Autodesk Inventor part; units mm, degrees
ref_plane "YZ Plane" through (0, 0, 0) normal (1, 0, 0) x (0, 1, 0)
ref_plane "XZ Plane" through (0, 0, 0) normal (0, 1, 0) x (-1, 0, 0)
ref_plane "XY Plane" through (0, 0, 0) normal (0, 0, 1) x (1, 0, 0)
sketch "Sketch1" plane through (0, 0, 0) normal (0, 0, 1) x (1, 0, 0)
  line L0 (40.11, 59.8927) -> (-34.89, 59.8927)
  line L1 (-34.89, 59.8927) -> (-34.89, -60.1073)
  line L2 (-34.89, -60.1073) -> (40.11, -60.1073)
  line L3 (-52.89, 89.8927) -> (68.11, 89.8927)
  line L4 (68.11, -90.1073) -> (-52.89, -90.1073)
  line L5 (-64.89, -78.1073) -> (-64.89, 77.8927)
  line L6 (80.11, 47.3927) -> (91.11, 47.3927)
  line L7 (95.11, 43.3927) -> (95.11, 36.3927)
  line L8 (91.11, 32.3927) -> (80.11, 32.3927)
  line L9 (115.11, -0.1073) -> (-34.89, -0.1073) construction
  line L10 (80.11, -47.6073) -> (91.11, -47.6073)
  line L11 (95.11, -43.6073) -> (95.11, -36.6073)
  line L12 (91.11, -32.6073) -> (80.11, -32.6073)
  line L13 (80.11, 77.8927) -> (80.11, 47.3927)
  line L14 (80.11, -47.6073) -> (80.11, -78.1073)
  arc A0 (95.11, 43.3927) -> (91.11, 47.3927) centre (91.11, 43.3927) ccw
  arc A1 (91.11, 32.3927) -> (95.11, 36.3927) centre (91.11, 36.3927) ccw
  arc A2 (95.11, -36.6073) -> (91.11, -32.6073) centre (91.11, -36.6073) ccw
  arc A3 (91.11, -47.6073) -> (95.11, -43.6073) centre (91.11, -43.6073) ccw
  arc A4 (80.11, 77.8927) -> (68.11, 89.8927) centre (68.11, 77.8927) ccw
  arc A5 (68.11, -90.1073) -> (80.11, -78.1073) centre (68.11, -78.1073) ccw
  arc A6 (-64.89, -78.1073) -> (-52.89, -90.1073) centre (-52.89, -78.1073) ccw
  arc A7 (-52.89, 89.8927) -> (-64.89, 77.8927) centre (-52.89, 77.8927) ccw
  line L15 (44.11, 19.8927) -> (76.11, 19.8927)
  line L16 (76.11, -20.1073) -> (44.11, -20.1073)
  line L17 (80.11, 32.3927) -> (80.11, 23.8927)
  line L18 (80.11, -24.1073) -> (80.11, -32.6073)
  line L19 (40.11, -60.1073) -> (40.11, -24.1073)
  line L20 (40.11, 23.8927) -> (40.11, 59.8927)
  arc A8 (76.11, 19.8927) -> (80.11, 23.8927) centre (76.11, 23.8927) ccw
  arc A9 (40.11, 23.8927) -> (44.11, 19.8927) centre (44.11, 23.8927) ccw
  arc A10 (44.11, -20.1073) -> (40.11, -24.1073) centre (44.11, -24.1073) ccw
  arc A11 (80.11, -24.1073) -> (76.11, -20.1073) centre (76.11, -24.1073) ccw
  line L21 (211.9676, -294.2124) -> (139.9676, -294.2124)
  line L22 (135.9676, -414.2124) -> (215.9676, -414.2124)
  line L23 (139.9676, -334.2124) -> (211.9676, -334.2124)
  line L24 (215.9676, -374.2124) -> (135.9676, -374.2124)
  line L25 (215.9676, -414.2124) -> (215.9676, -374.2124)
  line L26 (135.9676, -298.2124) -> (135.9676, -330.2124)
  line L27 (135.9676, -374.2124) -> (135.9676, -414.2124)
  line L28 (226.9676, -306.7124) -> (215.9676, -306.7124)
  line L29 (215.9676, -321.7124) -> (226.9676, -321.7124)
  line L30 (230.9676, -317.7124) -> (230.9676, -310.7124)
  line L31 (215.9676, -330.2124) -> (215.9676, -321.7124)
  line L32 (215.9676, -306.7124) -> (215.9676, -298.2124)
  arc A12 (230.9676, -310.7124) -> (226.9676, -306.7124) centre (226.9676, -310.7124) ccw
  arc A13 (226.9676, -321.7124) -> (230.9676, -317.7124) centre (226.9676, -317.7124) ccw
  arc A14 (211.9676, -334.2124) -> (215.9676, -330.2124) centre (211.9676, -330.2124) ccw
  arc A15 (135.9676, -330.2124) -> (139.9676, -334.2124) centre (139.9676, -330.2124) ccw
  arc A16 (139.9676, -294.2124) -> (135.9676, -298.2124) centre (139.9676, -298.2124) ccw
  arc A17 (215.9676, -298.2124) -> (211.9676, -294.2124) centre (211.9676, -298.2124) ccw
  point P0 (95.11, 32.3927)
  point P1 (95.11, 47.3927)
  point P2 (87.61, 39.8927)
  point P3 (87.61, -40.1073)
  point P4 (95.11, -32.6073)
  point P5 (95.11, -47.6073)
  point P6 (87.61, -40.1073)
  point P7 (135.9676, -294.2124)
  point P8 (135.9676, -334.2124)
  point P9 (230.9676, -306.7124)
  dimension "d22" = 75
  dimension "d23" = 120
  dimension "d24" = 30
  dimension "d25" = 15
  dimension "d26" = 15
  dimension "d27" = 80
  dimension "d28" = 4
  dimension "d29" = 4
  dimension "d30" = 12
  dimension "d31" = 40
  dimension "d32" = 4
  dimension "d33" = 7.5
  dimension "d34" = 7.5
  dimension "d52" = 80
  dimension "d53" = 120
  dimension "d54" = 40
  dimension "d55" = 40
  dimension "d56" = 15
  dimension "d58" = 15
  dimension "d59" = 12.5
  dimension "d60" = 12.5
  dimension "d61" = 4
  dimension "d62" = 40
  dimension "d63" = 15
extrude "Extrusion1" add sketch "Sketch1" along normal blind 5 contours L0 L1 L2 L19 A10 L16 A11 L18 L12 A2 L11 A3 L10 L14 A5 L4 A6 L5 A7 L3 A4 L13 L6 A0 L7 A1 L8 L17 A8 L15 A9 L20
sketch "Sketch3" plane through (0, 0, 5) normal (0, 0, 1) x (1, 0, 0)
  line L0 (95.11, 36.3927) -> (95.11, 43.3927)
  line L1 (95.11, -43.6073) -> (95.11, -36.6073)
  line L2 (91.11, 47.3927) -> (80.11, 47.3927)
  point P0 (0, 0)
  point P1 (87.61, 39.8927)
  point P2 (87.61, -40.1073)
  dimension "d35" = 7.5
  dimension "d36" = 7.5
  dimension "d37" = 80
  dimension "d38" = 7.5
hole "Hole1" at (87.61, 39.8927, 5) at (87.61, -40.1073, 5) direction (0, 0, -1) diameter 7 end through all
sketch "Sketch4" plane through (0, 0, 5) normal (0, 0, 1) x (1, 0, 0)
  line L0 (-64.89, 77.8927) -> (-64.89, -78.1073)
  line L1 (-64.89, -0.1073) -> (63.4668, -0.1073) construction
  line L2 (-52.89, -90.1073) -> (68.11, -90.1073)
  line L3 (68.11, 89.8927) -> (-52.89, 89.8927)
  point P0 (0, 0)
  point P1 (-49.89, 74.8927)
  point P2 (-49.89, -75.1073)
  point P3 (55.11, -75.1073)
  point P4 (55.11, 74.8927)
  dimension "d64" = 15
  dimension "d65" = 15
  dimension "d66" = 105
  dimension "d74" = 15
hole "Hole2" at (-49.89, 74.8927, 5) at (-49.89, -75.1073, 5) at (55.11, -75.1073, 5) at (55.11, 74.8927, 5) direction (0, 0, -1) diameter 7 end through all
sketch "Sketch5" plane through (0, 0, 5) normal (0, 0, 1) x (1, 0, 0)
  line L0 (76.11, -20.1073) -> (44.11, -20.1073)
  line L1 (40.11, -24.1073) -> (40.11, -60.1073)
  point P0 (0, 0)
  point P1 (60.11, -40.1073)
  dimension "d75" = 20
  dimension "d76" = 20
hole "Hole3" at (60.11, -40.1073, 5) direction (0, 0, -1) diameter 2 depth 1
equation "\"d59\" = d60"
properties part number "MarcoBC" material "MDF Medium Density Fiberboard"
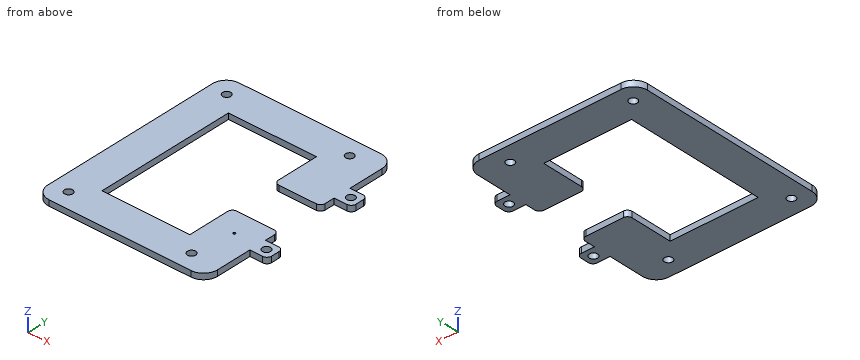
Here's how the part is built. I have some questions about the finished solid (model axes, mm). Give positions to 0.01 mm unless a question says otherwise; leave off trailing zeros. Order: outer loops, then holes, each group sorted by start corner. A loop starts at its lowest first (then second) coordinate and runs counter-clockwise, first axis right, second up. Notation, with made-up numbers: M 26,-1.75 L 60,-1.75 A33 ccw 60,26.25 Z; hole C 13.5,12 d2. An arc over 180 degrees is marked long. Answer as a JSON object with one key per item and string values. Group by question number.
1) Please list where these lines run through material, in increasing order: L1, parallel to Y at x = 55.11, z = 3.25; L2, parallel to Y at x = 60.11, z = 4.6; L3, parallel to Y at x = 31, z = 0.7. Write a range as [from, to].
2) I'm going to push flat-ended pins straight in: pin 1 Ø6 at (x, y) = (-29, -28.5) entering from +Z; pin 2 Ø8 at (x, y) = (39.5, -38.5) entering from +Z; pin 3 Ø1.5 at (x, z) = (86.5, 1.5) entering from -Y; pin 4 Ø3 at (x, z) = (75.5, 2.5) entering from -Y. Where does each tip first touch, or does it pass through?
3) Suppose I cut it at B-B, the plane x = -11. Write out the boundary of the cut face in (y, z), plus the area to 3 significant figures.
4) Suppose I cut it at C-C, the plane x = -49.89. Write out the boundary of the cut face in (y, z).
5) Suppose I cut it at A-A, the plane x = 55.11. Write out the boundary of the cut face in (y, z), plus the area to 3 significant figures.
6) Suppose I cut it at D-D, the plane x = 87.61. Write out the boundary of the cut face in (y, z).
Results found:
{
 "1": {"L1": "[-90.11, -78.61], [-71.61, -20.11], [19.89, 71.39], [78.39, 89.89]", "L2": "[-90.11, -41.11], [-39.11, -20.11], [19.89, 89.89]", "L3": "[-90.11, -60.11], [59.89, 89.89]"},
 "2": {"pin 1": "through", "pin 2": "z = 5", "pin 3": "y = -47.61", "pin 4": "y = -88.56"},
 "3": {"outline": "M -90.11,0 L -60.11,0 L -60.11,5 L -90.11,5 Z; M 59.89,0 L 89.89,0 L 89.89,5 L 59.89,5 Z", "area": "300 mm²"},
 "4": {"outline": "M -90.11,0 L -78.61,0 L -78.61,5 L -90.11,5 Z; M -71.61,0 L 71.39,0 L 71.39,5 L -71.61,5 Z; M 78.39,0 L 89.89,0 L 89.89,5 L 78.39,5 Z"},
 "5": {"outline": "M -90.11,0 L -78.61,0 L -78.61,5 L -90.11,5 Z; M -71.61,0 L -20.11,0 L -20.11,5 L -71.61,5 Z; M 19.89,0 L 71.39,0 L 71.39,5 L 19.89,5 Z; M 78.39,0 L 89.89,0 L 89.89,5 L 78.39,5 Z", "area": "630 mm²"},
 "6": {"outline": "M -47.61,0 L -43.61,0 L -43.61,5 L -47.61,5 Z; M -36.61,0 L -32.61,0 L -32.61,5 L -36.61,5 Z; M 32.39,0 L 36.39,0 L 36.39,5 L 32.39,5 Z; M 43.39,0 L 47.39,0 L 47.39,5 L 43.39,5 Z"}
}
